Source: three-view drawing plus pictorial views. Frame: mm from the lowest corner of the part. Coordinates: 2 decimals unless noted, no trailing zeros. Write each loop counter-clockwise with the first axis right and the second up, starting at its lowest first coordinate (ties: lowest second). Pieces come first, ordered by that corner, then holes. Notation, with made-up numbers: (42, 46) - (80, 46) arc R18 ccw to (80, 66) - close; hole circle Ø2 at (61.25, 31.25). An arc over 180 degrees is marked (long way). Answer as a JSON object with one key per item and string values. Group by question number.
Item 1: Section C-C on x = 68.5. Return loops of the section in (y, z).
Item 2: First-contact query: pin 1 Ø4 at (x, z) = (32, 5) entering from -Y; pin 2 Ø2.5 at (y, z) = (2.5, 114.5) entering from -X; pin 3 Ø2.5 at (y, z) = (3, 65) entering from -X. Flat tips, straight axial feed; report the tip coordinate or a pass-through.
Item 3: Line query: line 1 along Z through (x, y) = (58.5, 3.85); line 2 along Z through (x, y) = (32, 1.7); line 3 along X through (y, z) = (3.1, 145). Output: solid intervals per line, ascending. Write a range as from..to.
Item 4: Section A-A on x = 24. Return loops of the section in (y, z), and give its area (3 significant figures).
Item 5: Section D-D on z = 72.5. Return loops of the section in (x, y), and give its area (3 significant figures).
Item 6: Section B-B on y = 1.5. State how many separate pieces and enclosed holes the cut face has, and give its area (3 significant figures).
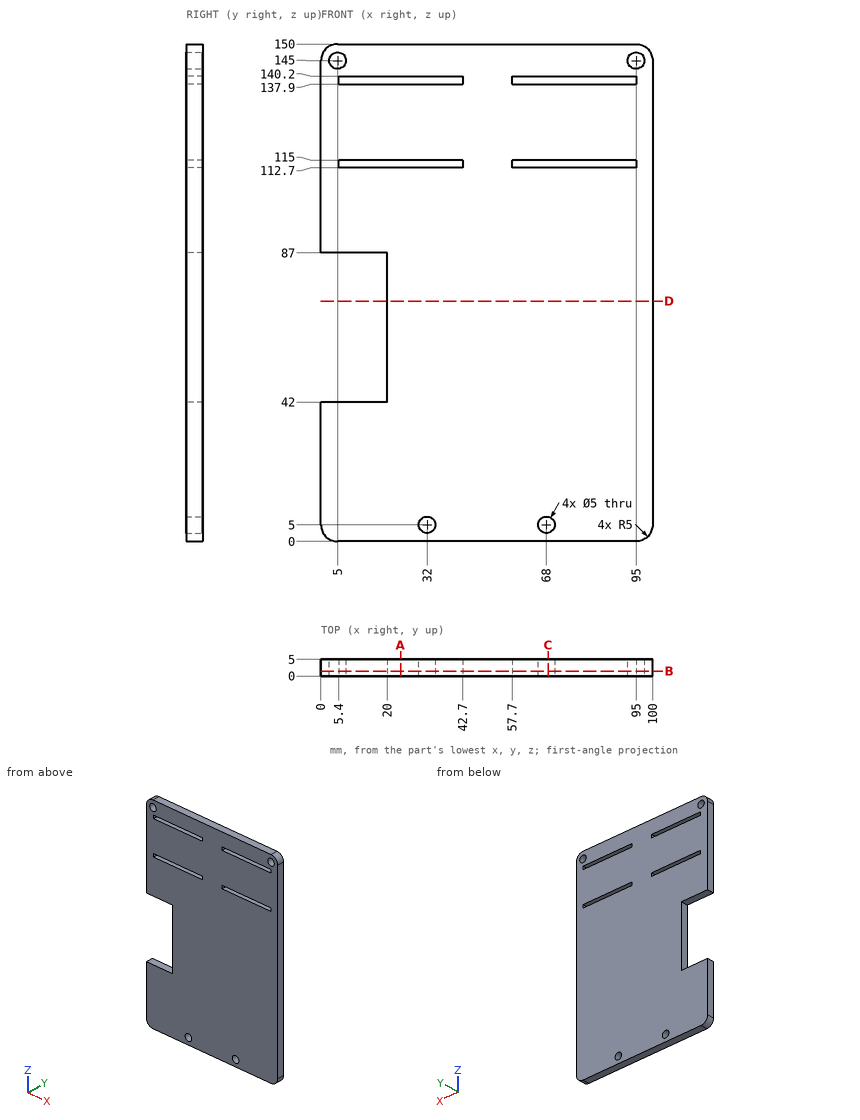
Checks:
{
 "1": {"outline": "(0, 0) - (5, 0) - (5, 2.55) - (0, 2.55) - close; (0, 7.45) - (5, 7.45) - (5, 112.7) - (0, 112.7) - close; (0, 115) - (5, 115) - (5, 137.9) - (0, 137.9) - close; (0, 140.2) - (5, 140.2) - (5, 150) - (0, 150) - close"},
 "2": {"pin 1": "through", "pin 2": "x = 0", "pin 3": "x = 20"},
 "3": {"line 1": "0..112.7, 115..137.9, 140.2..150", "line 2": "0..2.5, 7.5..112.7, 115..137.9, 140.2..150", "line 3": "0..2.5, 7.5..92.5, 97.5..100"},
 "4": {"outline": "(0, 0) - (5, 0) - (5, 112.7) - (0, 112.7) - close; (0, 115) - (5, 115) - (5, 137.9) - (0, 137.9) - close; (0, 140.2) - (5, 140.2) - (5, 150) - (0, 150) - close", "area": "727 mm^2"},
 "5": {"outline": "(20, 0) - (100, 0) - (100, 5) - (20, 5) - close", "area": "400 mm^2"},
 "6": {"separate pieces": "1", "enclosed holes": "8", "area": "13,700 mm^2"}
}
